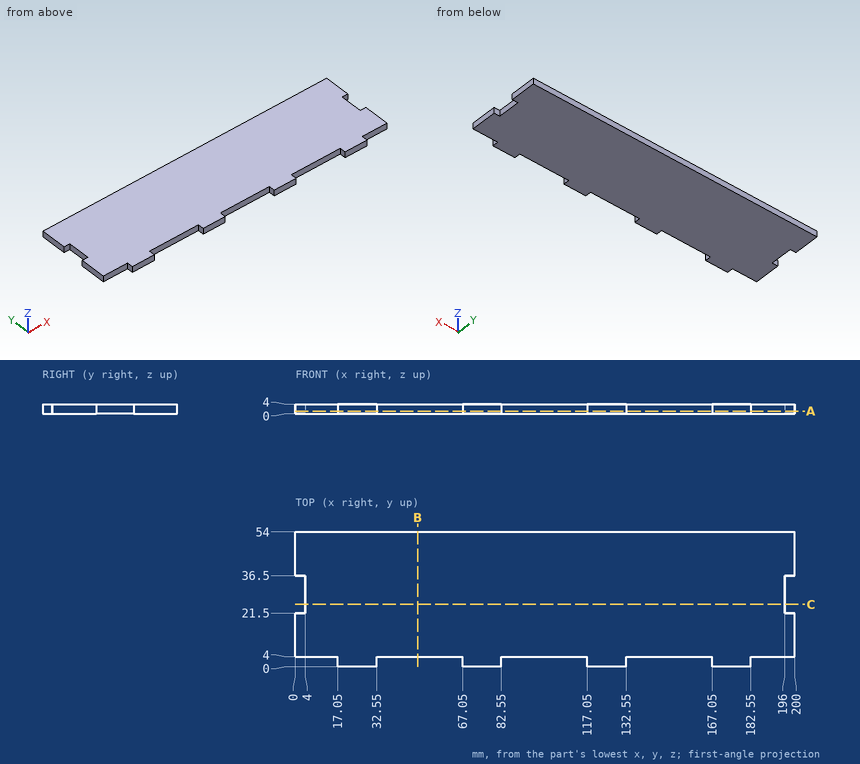
Input: dimensioned drawing with shaded views. Units: mm. Origin: part minimum x, y, z. Coordinates: 2 decimals unless noted, no trailing zeros. Loops run counter-clockwise (first coordinate to the right, second up) from the corner with the lowest first, then second, coordinate; pieces in that order, holes last. Notation, with made-up numbers: (58, 44) -> (82, 44) arc R16 ccw to (82, 50) -> close; hole circle Ø6 at (67, 5). An arc over 180 degrees is marked (long way). One line per item, written item: value. Start each with the question number.
Q1. Section query B-B, the plane x = 49. Return the cut outline in (y, z), and give its area (3 significant figures).
Q2. Section query A-A, the plane z = 1.15. Return the cut outline in (x, y), and give its area (3 significant figures).
Q3. Contact query for flat-ended pins moving along their axis: P1, Ø2, axis at x = 2, z = 1.5, coming from the -Y side; P2, Ø2, axis at y = 2, z = 2.5, coming from the +X side; P3, Ø1.2, axis at y = 1.5, z = 2.5, coming from the -X side. Output: stop coordinate, or through.
Q4. Line query: line 1 along X through (y, z) = (23.5, 2.7); line 2 along Y through (x, z) = (155.5, 1). Output: solid intervals per line, ascending.
Q5. Section query C-C, the plane y = 25. Return the cut outline in (x, z), and give its area (3 significant figures).
Results:
1. outline: (4, 0) -> (54, 0) -> (54, 4) -> (4, 4) -> close
1. area: 200 mm^2
2. outline: (0, 4) -> (17.05, 4) -> (17.05, 0) -> (32.55, 0) -> (32.55, 4) -> (67.05, 4) -> (67.05, 0) -> (82.55, 0) -> (82.55, 4) -> (117.05, 4) -> (117.05, 0) -> (132.55, 0) -> (132.55, 4) -> (167.05, 4) -> (167.05, 0) -> (182.55, 0) -> (182.55, 4) -> (200, 4) -> (200, 21.5) -> (196, 21.5) -> (196, 36.5) -> (200, 36.5) -> (200, 54) -> (0, 54) -> (0, 36.5) -> (4, 36.5) -> (4, 21.5) -> (0, 21.5) -> close
2. area: 10,100 mm^2
3. P1: y = 4
3. P2: x = 182.55
3. P3: x = 17.05
4. line 1: 4 to 196
4. line 2: 4 to 54
5. outline: (4, 0) -> (196, 0) -> (196, 4) -> (4, 4) -> close
5. area: 768 mm^2
